Design review of the part built by this model. Coordinates are the model's own, in mm. Face numbers are marked on the shaded views. A direction names the side the tool comes from. Round coordinates to 2 decimals unless told otherwise and drop trailing zeros. Loops run counter-clockwise (first coordinate to the right, second up) from the corner with the lowest first, then second, coordinate; pieces in that order, holes last. Notation, with made-up numbers: (-24, -2.5) -> (32, -2.5) arc R16 ccw to (32, 21.5) -> close; hole circle Ø11 at (15.5, 63.5). An arc over 180 degrees is marked (long way). Write each question's results on one line, items separated by ' | '. Start each with the question number.
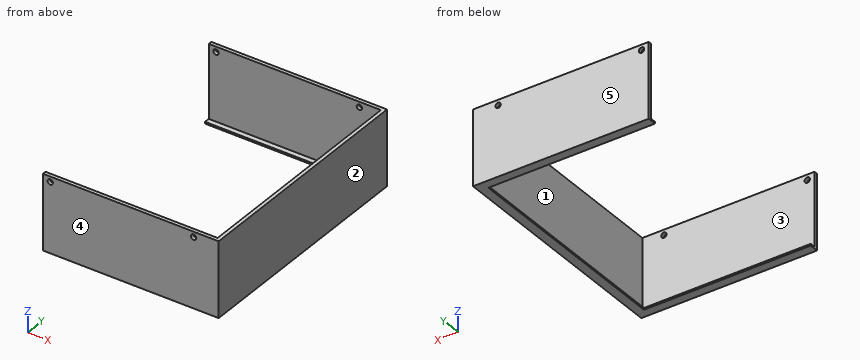
from build123d import *

# Parameters (mm, degrees)
SKETCH1_W           = 98
SKETCH1_H           = 6
SKETCH1_R           = 1.5
BOSS_EXTRUDE1_DEPTH = 2
SKETCH2_W           = 2
SKETCH2_H           = 6
BOSS_EXTRUDE2_DEPTH = 130
SKETCH3_W           = 98
SKETCH3_H           = 6
SKETCH3_R           = 1.5
BOSS_EXTRUDE3_DEPTH = 2
BOSS_EXTRUDE4_DEPTH = 35
BOSS_EXTRUDE5_DEPTH = 1


with BuildPart() as part:
    # Sketch1 → Boss-Extrude1 (new body)
    with BuildSketch(Plane(origin=(0, 0, 0), x_dir=(1, 0, 0), z_dir=(0, 1, 0))):
        with Locations((45, 0)):
            Rectangle(SKETCH1_W, SKETCH1_H)
        with Locations(Location((0, 0, 0), (0, 0, 270))):
            Circle(SKETCH1_R, mode=Mode.SUBTRACT)
        with Locations(Location((80, 0, 0), (0, 0, 270))):
            Circle(SKETCH1_R, mode=Mode.SUBTRACT)
    extrude(amount=BOSS_EXTRUDE1_DEPTH)

    # Sketch2 → Boss-Extrude2 (add)
    with BuildSketch(Plane(origin=(0, 2, 0), x_dir=(1, 0, 0), z_dir=(0, 1, 0))):
        with Locations((93, 0)):
            Rectangle(SKETCH2_W, SKETCH2_H)
    extrude(amount=BOSS_EXTRUDE2_DEPTH)

    # Sketch3 → Boss-Extrude3 (add)
    with BuildSketch(Plane(origin=(0, 132, 0), x_dir=(1, 0, 0), z_dir=(0, 1, 0))):
        with Locations((45, 0)):
            Rectangle(SKETCH3_W, SKETCH3_H)
        with Locations(Location((0, 0, 0), (0, 0, 270))):
            Circle(SKETCH3_R, mode=Mode.SUBTRACT)
        with Locations(Location((80, 0, 0), (0, 0, 270))):
            Circle(SKETCH3_R, mode=Mode.SUBTRACT)
    extrude(amount=BOSS_EXTRUDE3_DEPTH)

    # Sketch4 → Boss-Extrude4 (add)
    with BuildSketch(Plane(origin=(0, 0, -3), x_dir=(-1, 0, 0), z_dir=(0, 0, -1))):
        Polygon((4, 0), (-92, 0), (-94, 0), (-94, 134), (-92, 134), (4, 134), (4, 132), (-92, 132), (-92, 2), (4, 2), align=None)
    extrude(amount=BOSS_EXTRUDE4_DEPTH)

    # Sketch5 → Boss-Extrude5 (add)
    with BuildSketch(Plane(origin=(0, 0, -38), x_dir=(-1, 0, 0), z_dir=(0, 0, -1))):
        Polygon((4, 0), (-94, 0), (-94, 5), (-94, 126), (-94, 134), (4, 134), (4, 129), (-89, 129), (-89, 5), (4, 5), align=None)
    extrude(amount=BOSS_EXTRUDE5_DEPTH)


solid = part.part
1) For the marked faces 1 and 2, list the 3-axis set-ups (+Z, -Z, +X, -X, +Y, -Y) from which the entire face can be reached by the end or side of a thin tool; tool diameter is ignored.
2) The part is to be moulded in two halves that separate along Y. For the marked faces 3, 4 and 5, say which applies: +Y half, -Y half, draft (parallel to the pull), parting line (faces both ways), or undercut.
3) Insertion check: pin 1 (4 mm diameter, centred on y = 77.5, z = -20.5, fed in from -X); pin 2 (3 mm diameter, centred on x = 56, z = -16.5, fed in from -Y); pin 3 (2.5 mm diameter, centred on x = 80, z = 0, fed in from -Y); pin 4 (0.8 mm diameter, centred on y = 63, z = -38.5, fed in from -X). Each pin has a flat end and moves straight along its axis. Give the tip position at first contact, or say it passes through.
4) Take a section at B-B (x = 0). Write out the cut boundary in (y, z), plus the area to 3 significant figures.
5) Take a section at D-D (z = -34). Write out the cut boundary in (x, y), plus the area to 3 significant figures.
6) Take a section at C-C (z = 0). Write out the cut boundary in (x, y).
7) To check wall thickness, follow line 1 (X direction, y = 1.55, z = 0); line 2 (Y direction, x = 36.5, z = -4); line 3 (Z direction, x = 80, y = 1). State the ranges of each line that lie inside material, in increasing order. Write a range as from..to.
8) Take a section at A-A (x = 61.5). Write out the cut boundary in (y, z).
Geometry check:
1) face 1: +Z, -X | face 2: +Z, -Z, +X, +Y, -Y
2) face 3: undercut | face 4: -Y half | face 5: +Y half
3) pin 1: stops at x = 92 | pin 2: stops at y = 0 | pin 3: passes through | pin 4: stops at x = 89
4) outline: (0, -39) -> (5, -39) -> (5, -38) -> (2, -38) -> (2, -1.5) -> (0, -1.5) -> close; (0, 1.5) -> (2, 1.5) -> (2, 3) -> (0, 3) -> close; (129, -39) -> (134, -39) -> (134, -1.5) -> (132, -1.5) -> (132, -38) -> (129, -38) -> close; (132, 1.5) -> (134, 1.5) -> (134, 3) -> (132, 3) -> close | area: 162 mm^2
5) outline: (-4, 0) -> (94, 0) -> (94, 134) -> (-4, 134) -> (-4, 132) -> (92, 132) -> (92, 2) -> (-4, 2) -> close | area: 652 mm^2
6) outline: (-4, 0) -> (-1.5, 0) -> (-1.5, 2) -> (-4, 2) -> close; (-4, 132) -> (-1.5, 132) -> (-1.5, 134) -> (-4, 134) -> close; (1.5, 0) -> (78.5, 0) -> (78.5, 2) -> (1.5, 2) -> close; (1.5, 132) -> (78.5, 132) -> (78.5, 134) -> (1.5, 134) -> close; (81.5, 0) -> (94, 0) -> (94, 134) -> (81.5, 134) -> (81.5, 132) -> (92, 132) -> (92, 2) -> (81.5, 2) -> close
7) line 1: x = -4..-1.5, 1.5..78.5, 81.5..94 | line 2: y = 0..2, 132..134 | line 3: z = -39..-1.5, 1.5..3
8) outline: (0, -39) -> (5, -39) -> (5, -38) -> (2, -38) -> (2, 3) -> (0, 3) -> close; (129, -39) -> (134, -39) -> (134, 3) -> (132, 3) -> (132, -38) -> (129, -38) -> close
